Autodesk Inventor part; units mm, degrees
ref_plane "Work Plane1" through (104.775, 0, 0) normal (0, 0, -1) x (1, 0, 0)
ref_plane "YZ Plane" through (0, 0, 0) normal (1, 0, 0) x (0, 1, 0)
ref_plane "XZ Plane" through (0, 0, 0) normal (0, 1, 0) x (-1, 0, 0)
sketch "Sketch1" plane through (0, 0, 0) normal (0, 0, 1) x (1, 0, 0)
  line L0 (8, 0) -> (8, 1)
  line L1 (8, 1) -> (2.95, 1)
  line L2 (2.95, 1) -> (2.6433, 1)
  line L3 (0, 2) -> (0, 0.7217)
  line L4 (0, 0.7217) -> (0.95, 0.7217)
  line L5 (0.95, 0.7217) -> (1.3667, 0)
  line L6 (1.3667, 0) -> (8, 0)
  line L7 (0, 2) -> (0, 2)
  line L8 (0, 2) -> (1, 1)
  line L9 (2.6433, 1) -> (1, 1)
  line L10 (2.95, 1) -> (1, 1) construction
  line L11 (1, 1) -> (1, 1)
  line L12 (-1.6, 0) -> (9.6, 0)
  line L13 (0, -0.4) -> (0, 2.4)
  dimension "d0" = 8
  dimension "d1" = 5.05
  dimension "d2" = 0.95
  dimension "d3" = 2
  dimension "d6" = 1
  dimension "d7" = 45
  dimension "d8" = 1.4434
  dimension "d9" = 60
  dimension "d10" = 4
  dimension "d11" = 2
  dimension "d12" = 0.3067
revolve "Body" add sketch "Sketch1" angle 360 about axis through (1.3667, 0, 0) along (1, 0, 0) contours L6 L5 L4 L3 L8 L9 L2 L1 L0
thread "Thread"
chamfer "Chamfer1" distance 0.3067 distance2 0.3067 1 edges at (8, -1, 0) measured on face at (8, 0.202, 0.5327)
ref_plane "Work Plane1" through (104.775, 0, 0) normal (0, 0, -1) x (1, 0, 0)
sketch "Sketch4" plane through (0, 0, 0) normal (-1, 0, 0) x (0, 0, 1)
  circle A0 centre (0, 0) radius 0.7217
  line L0 (0.625, -0.3608) -> (0, -0.7217)
  line L1 (0, -0.7217) -> (-0.625, -0.3608)
  line L2 (-0.625, -0.3608) -> (-0.625, 0.3608)
  line L3 (-0.625, 0.3608) -> (0, 0.7217)
  line L4 (0, 0.7217) -> (0.625, 0.3608)
  line L5 (0.625, 0.3608) -> (0.625, -0.3608)
  point P0 (0, 0)
  point P1 (0.625, 0.3608)
  point P2 (0.625, 0.3608)
  point P3 (0, 0.7217)
  point P4 (0, 0.7217)
  point P5 (-0.625, 0.3608)
  point P6 (-0.625, 0.3608)
  point P7 (0, -0.7217)
  point P8 (0, -0.7217)
extrude "Extrusion3" add sketch "Sketch4" against normal up to surface contours A0 L5 | L4 A0 | A0 L0 | L3 A0 | A0 L1 | L2 A0
equation "\"d17\" = -0.5 * SPD + 0.5 * GD"
equation "\"d18\" = GUL"
equation "\"d0\" = NLG"
equation "\"d1\" = GEL"
equation "\"d2\" = INTI"
equation "\"d3\" = GD"
equation "\"d6\" = KOH"
equation "\"d7\" = 0.5 * SEWI"
equation "\"d8\" = 1.1547 * SW"
equation "\"d10\" = KOD"
equation "\"d11\" = BDM"
equation "\"d12\" = GAL"
equation "\"NLG\" = 8"
equation "\"INTI\" = 0.95"
equation "\"GEL\" = 5.05"
equation "\"GAL\" = 0.61345 * PTC"
equation "\"KOH\" = 1"
equation "\"KOD\" = 4"
equation "\"GUL\" = 0.61345 * PTC"
equation "\"SPD\" = NND - 1.2269 * PTC"
equation "\"BDM\" = NND"
equation "\"GD\" = NND"
equation "\"SEWI\" = 90deg"
equation "\"SW\" = 1.25"
equation "\"TOA\" = 30deg"
equation "\"GD1\" = THREADDIA - 1.2269 * PTC"
equation "\"EPV\" = 3.2"
equation "\"THREADDIA\" = 3"
equation "\"PTC\" = 0.5"
equation "\"NND\" = 2"
equation "\"E0\" = 1.155 * SW"
properties part number "UNI 5933 - M3 x 8" material "Steel, Mild"
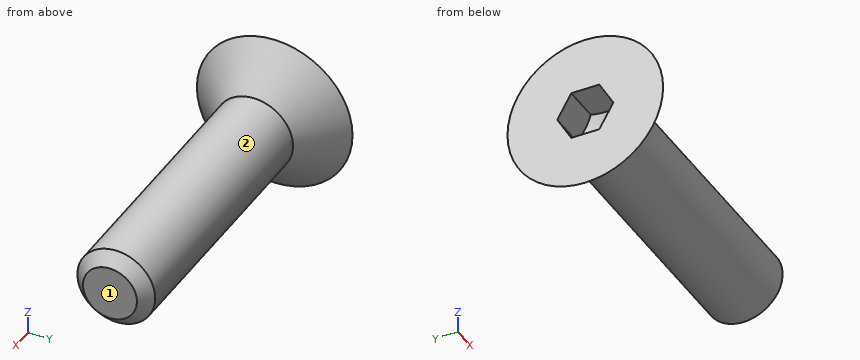
Could you check a few things on this model? Use its own coordinates, in mm. Face numbers are marked on the shaded views. A direction names the side the tool comes from. Round coordinates to 2 decimals unless told otherwise and drop trailing zeros. Write each loop counter-clockwise with the first axis right and the second up, starting at its lowest first coordinate (ties: lowest second). Pieces come first, ordered by that corner, then holes. Notation, with made-up numbers: (-36, 33) -> (-24, 33) arc R22 cw to (-24, 69) -> close; hole circle Ø5 at (33.25, 75). An arc over 180 degrees is marked (long way). Use a Markdown table: item, result.
1. If we section it at A-A (x = 1.75): List the corners of the cut face in (y, z) for me.
Answer key:
| item | result |
|---|---|
| outline | circle Ø2 at (0, 0) |
2. Please list where these lines run through material, in increasing order: probe 1 along X at (y, z) = (-0.15, -1.65); probe 2 along X at (y, z) = (-0.75, -0.5); probe 3 along Z at (x, y) = (5.75, 0.25).
Answer key:
| item | result |
|---|---|
| probe 1 | x = 0 to 0.34 |
| probe 2 | x = 0 to 7.79 |
| probe 3 | z = -0.97 to 0.97 |
3. Which directions (+Z, -Z, +X, -X, +Y, -Y) give clear straight access to the entire face, cutting with the end or side of a thin tool? Please do the marked faces 1 and 2.
Answer key:
| item | result |
|---|---|
| face 1 | +Z, -Z, +X, +Y, -Y |
| face 2 | +X |
4. For pin 1 Ø0.6 at (x, y) = (0.5, 0) entering from -Z; pin 2 Ø1.5 at (x, z) = (1, -1) entering from -Y; pin 3 Ø1 at (x, z) = (5.5, 0.5) entering from -Y, each with a flat end and sliding along its axis, tell me the tip position at first contact or that it passes through.
Answer key:
| item | result |
|---|---|
| pin 1 | stops at z = -1.8 |
| pin 2 | stops at y = -1.54 |
| pin 3 | stops at y = -1 |
